The listing builds one solid part. Answer for the finished solid, in the listing's coordinates (mm). Face numbers are marked on the shaded views. A direction names the side the tool comes from. Give positions to 0.01 mm unless a question says otherwise; leave off trailing zeros. Write each loop counter-clockwise with the first axis right and the second up, starting at its lowest first coordinate (ties: lowest second). Pieces come first, ordered by that corner, then holes. Notation, with made-up numbers: (-28, 36) -> (4, 36) arc R20 ccw to (4, 45) -> close; hole circle Ø4 at (62, -13). An arc over 180 degrees is marked (long way). One line per question, with ' | ' between items.
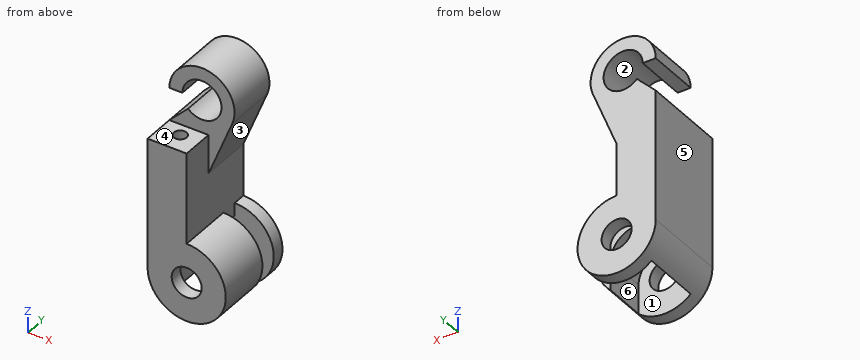
Autodesk Inventor part; units mm, degrees
ref_plane "YZ Plane" through (0, 0, 0) normal (1, 0, 0) x (0, 1, 0)
ref_plane "XZ Plane" through (0, 0, 0) normal (0, 1, 0) x (-1, 0, 0)
ref_plane "XY Plane" through (0, 0, 0) normal (0, 0, 1) x (1, 0, 0)
sketch "スケッチ1" plane through (0, 0, 0) normal (0, 1, 0) x (-1, 0, 0)
  circle A0 centre (0, 0) radius 1.15
  circle A1 centre (0, 0) radius 2
  circle A2 centre (0, 0) radius 3
  line L0 (0, 0) -> (0, 3)
  line L1 (-2, 0) -> (2, 0)
  line L2 (2, 0) -> (2, -3)
  line L3 (2, -3) -> (-2, -3)
  line L4 (-2, -3) -> (-2, 0)
  line L5 (0, 0) -> (3, 0)
  line L6 (3, 0) -> (3, 3)
  line L7 (3, 3) -> (0, 3)
  line L8 (0, 3) -> (0, 0)
  point P0 (-2, -2.2361)
  point P1 (0, 2)
  point P2 (2, -2.2361)
  dimension "d1" = 4
  dimension "d2" = 6
  dimension "d0" = 2.3
extrude "押し出し1" add sketch "スケッチ1" along normal blind 3.2 contours A1 L4 A2 L0
extrude "押し出し2" add sketch "スケッチ1" along normal blind 4.5 contours L5 A2 L2 | A1 L0 A2 L5 | A2 L7 L6
extrude "押し出し3" add sketch "スケッチ1" against normal blind 1 contours L1 A1 A0 | A0 L0 A1 L1 | A0 L1 A1 L0 | L2 A2 L4 A1 | L5 A2 L2 | A1 L0 A2 L5 | A1 L4 A2 L0 | A2 L7 L6
sketch "スケッチ2" plane through (0, 4.5, 0) normal (0, 1, 0) x (1, 0, 0)
  circle A0 centre (0, 0) radius 1.15
  circle A1 centre (0, 0) radius 2
  circle A2 centre (0, 0) radius 3
  line L0 (0, 0) -> (-3, 0)
  line L1 (-3, 0) -> (-3, -3)
  line L2 (-3, -3) -> (0, -3)
  line L3 (0, -3) -> (0, 0)
  dimension "d9" = 2.3
  dimension "d10" = 4
  dimension "d11" = 6
extrude "押し出し4" add sketch "スケッチ2" along normal blind 1 contours A0 L0 A1 L3 | A0 L3 A1 L0 | L0 A2 L3 A1 | A1 L3 A2 L0 | A2 L2 L1
sketch "スケッチ3" plane through (-3, -1, 3) normal (0, 0, 1) x (1, 0, 0)
  line L0 (0, 6.5) -> (0, 0)
  line L1 (3, 5.5) -> (3, 6.5)
  line L2 (0, 0) -> (3, 0)
  line L3 (3, 0) -> (3, 6.5)
  line L4 (3, 6.5) -> (0, 6.5)
  line L5 (0, 6.5) -> (0, 0)
  point P0 (3, 1)
extrude "押し出し5" add sketch "スケッチ3" along normal blind 7
sketch "スケッチ4" plane through (-3, -1, 10) normal (0, 0, 1) x (1, 0, 0)
  line L0 (4.15, 0) -> (1.85, 0)
  line L1 (3, 0) -> (1.5, 0)
  line L2 (1.5, 0) -> (1.5, 1.5)
  line L3 (1.5, 1.5) -> (3, 1.5)
  line L4 (3, 1.5) -> (3, 0)
  point P0 (3, 1)
  dimension "d16" = 1.5
  dimension "d17" = 1.5
hole "穴1" at (-1.5, 0.5, 10) direction (0, 0, -1) diameter 1 end through all
sketch "スケッチ5" plane through (0, 3.2, 3) normal (1, 0, 0) x (0, 0, -1)
  point P0 (3, -3.2)
sketch "スケッチ6" plane through (0, 5.5, 0) normal (0, 1, 0) x (1, 0, 0)
  line L0 (-3, -10) -> (0, -10)
  line L1 (-3, -10) -> (2, -10)
  line L2 (2, -10) -> (2, -15)
  line L3 (2, -15) -> (-3, -15)
  line L4 (-3, -15) -> (-3, -10)
  line L5 (2, -10) -> (-0.5, -10)
  line L6 (-0.5, -10) -> (-0.5, -12.5)
  line L7 (-0.5, -12.5) -> (2, -12.5)
  line L8 (2, -12.5) -> (2, -10)
  circle A0 centre (-0.5, -12.5) radius 2.5
  circle A1 centre (-0.5, -12.5) radius 1.5
  line L9 (-0.5, -12.5) -> (-3, -10)
  line L10 (-0.5, -12.5) -> (-3, -12.5)
  line L11 (0, -3) -> (0, -10)
  line L12 (-3, -10) -> (0, -10)
  line L13 (0, -10) -> (0, -7)
  line L14 (0, -7) -> (-3, -7)
  line L15 (-3, -7) -> (-3, -10)
  line L16 (0, -7) -> (1.8225, -11.5748)
  point P0 (0, 0)
  point P1 (-2, -12.5)
  point P2 (-1.5607, -11.4393)
  dimension "d25" = 5
  dimension "d26" = 5
  dimension "d27" = 2.5
  dimension "d28" = 2.5
  dimension "d29" = 3
  dimension "d30" = 3
extrude "押し出し6" add sketch "スケッチ6" against normal blind 4 contours L0 A0 L9 | A0 L7 A1 L6 | L0 L1 L16 A0 | L6 A1 L9 A0 | L10 A1 L7 A0 | L11 L16 L1
properties part number "srod1.1"
Item 1: Flat-ended cylindrical pins translate along their axes: pin 1 (1.1 mm diameter, centred on y = 3, z = -1, fed in from +X); pin 2 (1 mm diameter, centred on y = 2.5, z = 5, fed in from +X); pin 3 (1 mm diameter, centred on x = 2, y = 2, fed in from +Z). Find the tip coordinate at first contact, or state that the pin passes through.
Answers below:
pin 1: x = 2.97 | pin 2: x = 0 | pin 3: z = 14
Item 2: Find section B-B (x = -0.65). Write down the section's boundary in (y, z), then the cut area to 3 significant figures.
Answers below:
outline: (-1, -2.93) -> (0, -2.93) -> (0, -0.95) -> (-1, -0.95) -> close; (-1, 0.95) -> (0, 0.95) -> (0, 1.89) -> (4.5, 1.89) -> (4.5, 0.95) -> (5.5, 0.95) -> (5.5, 11.01) -> (1.5, 11.01) -> (1.5, 10) -> (-1, 10) -> close; (1.5, 13.99) -> (5.5, 13.99) -> (5.5, 15) -> (1.5, 15) -> close; (4.5, -2.93) -> (5.5, -2.93) -> (5.5, -0.95) -> (4.5, -0.95) -> close | area: 66.6 mm²
Item 3: Find section A-A (z = -0.75). Write down the section's boundary in (x, y).
Answers below:
outline: (-2.9, -1) -> (-0.87, -1) -> (-0.87, 0) -> (-2, 0) -> (-2, 4.5) -> (-0.87, 4.5) -> (-0.87, 5.5) -> (-2.9, 5.5) -> close; (0.87, -1) -> (2.9, -1) -> (2.9, 3.2) -> (2, 3.2) -> (2, 0) -> (0.87, 0) -> close; (0.87, 4.5) -> (2.9, 4.5) -> (2.9, 5.5) -> (0.87, 5.5) -> close
Item 4: Consider line 1 (X direction, y = 0.5, z = 8); line 2 (X direction, y = -0.8, z = 0); line 3 (Y direction, x = 1.7, z = -1.5). Determine where each line is inside the solid, lowest interval first. Write a range as [from, to].
Answers below:
line 1: [-3, -2], [-1, 0] | line 2: [-3, -1.15], [1.15, 3] | line 3: [-1, 0], [4.5, 5.5]
Item 5: A tool of negligible diameter and unlimited length cuts with its end or side. For the marked faces 5 and 6, from which of +Z, -Z, +X, -X, +Y, -Y can it reach the whole face along a straight path? Write none if from no direction.
Answers below:
face 5: +Z, -Z, -X, +Y, -Y | face 6: -Z
Item 6: Find section D-D (y = 2.75). Write down the section's boundary in (x, z), then the cut area to 3 significant figures.
Answers below:
outline: (-3, 0) arc R3 ccw to (-2, -2.24) -> (-2, 0) arc R2 cw to (2, 0) -> (2, -2.24) arc R3 ccw to (0, 3) -> (0, 7) -> (1.82, 11.57) arc R2.5 ccw (long way) to (-3, 12.5) -> (-2, 12.5) arc R1.5 cw (long way) to (-1.56, 11.44) -> (-3, 10) -> close | area: 47.9 mm²
Item 7: Find section C-C (z = 13.75). Write down the section's boundary in (x, y), then the cut area to 3 significant figures.
Answers below:
outline: (-2.67, 1.5) -> (-1.33, 1.5) -> (-1.33, 5.5) -> (-2.67, 5.5) -> close; (0.33, 1.5) -> (1.67, 1.5) -> (1.67, 5.5) -> (0.33, 5.5) -> close | area: 10.7 mm²
Item 8: Determine the mould class of the marked faces 1, 2, 3 and 4 for opening direction Z: pulls with the +Z half, pulls with the -Z half, needs draft (parallel to the pull), parting line crosses it, or undercut.
Answers below:
face 1: needs draft | face 2: undercut | face 3: undercut | face 4: pulls with the +Z half
